from build123d import *

# Parameters (mm, degrees)
F1_DEPTH = 19.05
F2_W     = 101.854
F2_H     = 19.304
F3_DEPTH = 25.4


# Not quite as in the source:
# - a feature names something its author has since deleted; it is built from what else it names


with BuildPart() as f1:
    # F0 (on Top) → F1 (new body)
    with BuildSketch(Plane.XY):
        Polygon((-69.3041831255, 0), (-69.3041831255, -150.0828219056), (1607.0958168745, -150.0828219056), (1607.0958168745, 129.3171780944), (1962.6958168745, 129.3171780944), (1962.6958168745, 332.5171780944), (1607.0958168745, 332.5171780944), (1607.0958168745, 611.9171780944), (-69.3041831255, 611.9171780944), align=None)
    extrude(amount=F1_DEPTH)

    # F2 (on face) → F3 (cut)
    with BuildSketch(Plane.XY.offset(19.05)):
        with Locations((464.2228168745, 532.6691780944)):
            Rectangle(F2_W, F2_H)
        with Locations((464.2228168745, -70.8348219056)):
            Rectangle(F2_W, F2_H)
        Polygon((-69.3041831255, 307.3549188137), (-69.3041831255, 224.8049188137), (-69.3041831255, 142.2549188137), (235.4958168745, 142.2549188137), (235.4958168745, 307.3549188137), align=None)
    extrude(amount=-F3_DEPTH, mode=Mode.SUBTRACT)


solid = f1.part
Part model, mm, in its own coordinate system. Round coordinates to 2 decimals unless told otherwise and drop trailing zeros. Write each loop counter-clockwise with the first axis right and the second up, starting at its lowest first coordinate (ties: lowest second). Pieces come first, ordered by that corner, then holes. Notation, with made-up numbers: M 52,72.5 L 60,72.5 A28 ccw 60,93.5 Z; hole C -17.5,88 d6. An arc over 180 degrees is marked long. Return JSON: item names as keys, results as strings. Group by question number.
(1) Saw through at C-C on x = 1818. Write the cut outline in (y, z), then the cut area to 3 significant figures.
(2) Saw through at A-A on z = 13.25. Write the cut outline in (x, y).
(3) Drill centre lines: probe 1 along Y at (x, z) = (492.5, 16); probe 2 along Y at (x, z) = (70.5, 11); probe 3 along X at (y, z) = (550.5, 11.75). Where is each one in solid material? Low to high.
(4) Saw through at B-B on y = 43. Write the cut outline in (x, z), then the cut area to 3 significant figures.
(5) Pin check, flat tips, straight feed: pin 1 Ø10 at (y, z) = (-20.5, 4) entering from +X; pin 2 Ø9.5 at (y, z) = (192, 5) entering from -X; pin 3 Ø9.5 at (x, z) = (1800.5, 12) entering from -Y. Stop position of each tip, or through.
Returned:
{
 "1": {"outline": "M 129.32,0 L 332.52,0 L 332.52,19.05 L 129.32,19.05 Z", "area": "3,870 mm²"},
 "2": {"outline": "M -69.3,-150.08 L 1607.1,-150.08 L 1607.1,129.32 L 1962.7,129.32 L 1962.7,332.52 L 1607.1,332.52 L 1607.1,611.92 L -69.3,611.92 L -69.3,307.35 L 235.5,307.35 L 235.5,142.25 L -69.3,142.25 Z; hole M 413.3,-80.49 L 515.15,-80.49 L 515.15,-61.18 L 413.3,-61.18 Z; hole M 413.3,523.02 L 515.15,523.02 L 515.15,542.32 L 413.3,542.32 Z"},
 "3": {"probe 1": "-150.08 to -80.49, -61.18 to 523.02, 542.32 to 611.92", "probe 2": "-150.08 to 142.25, 307.35 to 611.92", "probe 3": "-69.3 to 1607.1"},
 "4": {"outline": "M -69.3,0 L 1607.1,0 L 1607.1,19.05 L -69.3,19.05 Z", "area": "31,900 mm²"},
 "5": {"pin 1": "x = 1607.1", "pin 2": "x = 235.5", "pin 3": "y = 129.32"}
}
